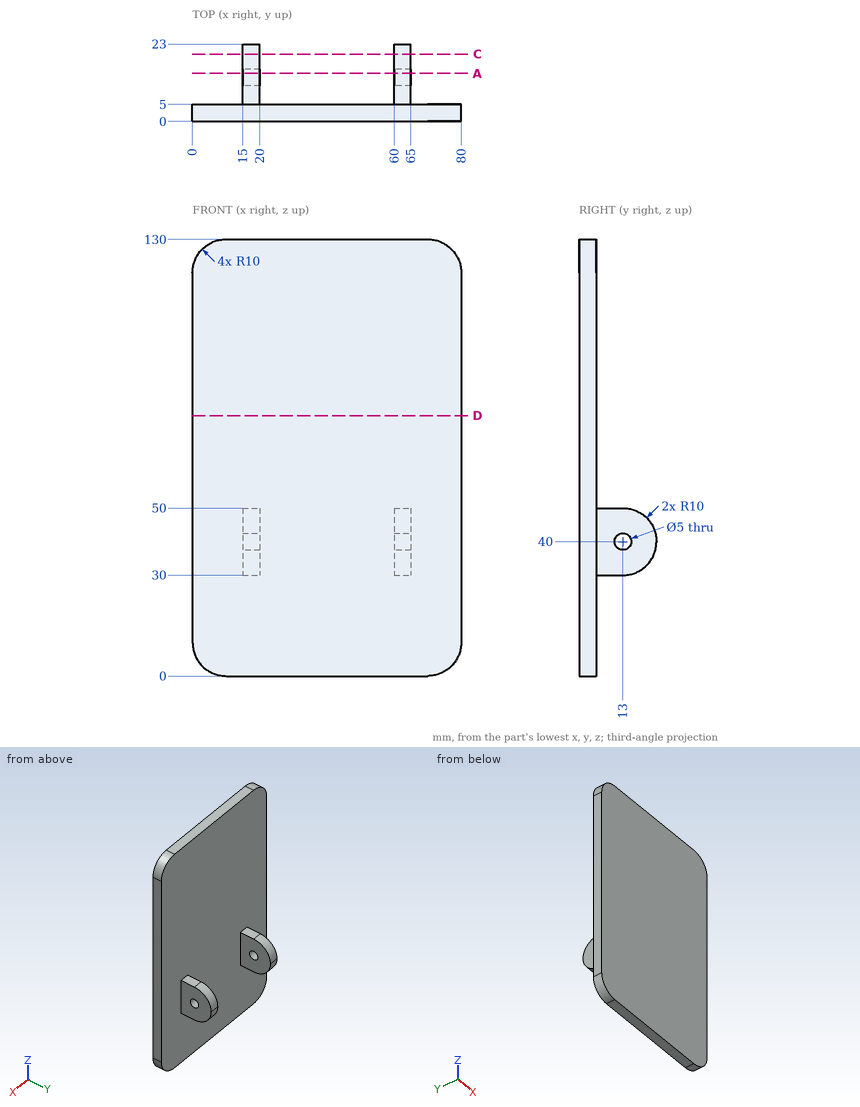
Answer from the drawing. Dimensions are ordinates in mm from the lowest x, y and z of the part. Give positions to 0.01 mm unless a question says otherwise; leave off trailing zeros. Order: outer loops, then holes, each group sorted by start corner. A loop starts at its lowest first (then second) coordinate and runs counter-clockwise, first axis right, second up. Notation, with made-up numbers: (-9, 67.5) - (10, 67.5) arc R17 ccw to (10, 93.5) - close; hole circle Ø11 at (88.25, 19.5). An arc over 180 degrees is marked (long way). One line per item, written item: value. Start each with the question number.
1) Find the intervals of material crossed by L1, parallel to Y at x = 61, z = 40; L2, parallel to X at y = 18, z = 39; L3, parallel to Y at x = 14, z = 74.5, in increasing order.
2) A cutting plane is placed at A-A on y = 14.25. Give the vertices of the cut face in (x, z) (1 decimal).
3) Given pin 1 Ø2.5 at (x, y) = (18, 9.5) entering from -Z; pin 2 Ø4 at (x, y) = (62, 10.5) entering from +Z; pin 3 Ø9 at (y, z) = (11.5, 45) entering from -X, each flat-ended and moving along its own axis, determine where each tip first touches the part or whether it passes through.
4) A cutting plane is placed at C-C on y = 20. Give the vertices of the cut face in (x, z).
5) A cutting plane is placed at D-D on z = 77.5. Give the vertices of the cut face in (x, y), then the cut area to 3 significant figures.
Answer sheet:
1. L1: y = 0 to 10.5, 15.5 to 23
1. L2: x = 15 to 20, 60 to 65
1. L3: y = 0 to 5
2. outline: (15, 30.1) - (20, 30.1) - (20, 37.8) - (15, 37.8) - close; (15, 42.2) - (20, 42.2) - (20, 49.9) - (15, 49.9) - close; (60, 30.1) - (65, 30.1) - (65, 37.8) - (60, 37.8) - close; (60, 42.2) - (65, 42.2) - (65, 49.9) - (60, 49.9) - close
3. pin 1: stops at z = 30
3. pin 2: stops at z = 50
3. pin 3: stops at x = 15
4. outline: (15, 32.86) - (20, 32.86) - (20, 47.14) - (15, 47.14) - close; (60, 32.86) - (65, 32.86) - (65, 47.14) - (60, 47.14) - close
5. outline: (0, 0) - (80, 0) - (80, 5) - (0, 5) - close
5. area: 400 mm2
